Job drawing, mm, ordinate dimensions from the low corner. One solid piece. Coordinates: 2 decimals unless noted, no trailing zeros. Write each loop counter-clockwise with the first axis right and the second up, starting at its lowest first coordinate (ties: lowest second). Pieces come first, ordered by that corner, then holes.
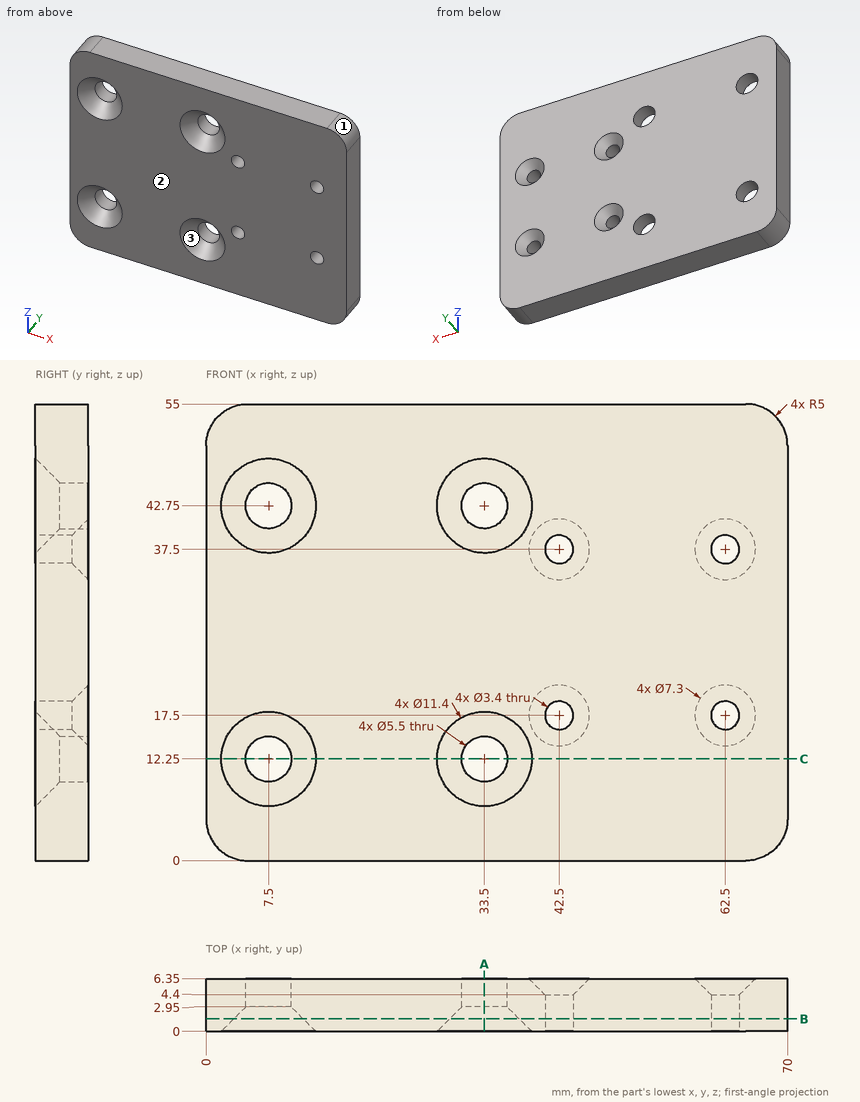
1. Saw through at C-C on z = 12.25. List the corners of the cut face in (x, y), plus the area to 3 significant figures.
Computed values:
outline: (0, 0) - (1.8, 0) - (4.75, 2.95) - (4.75, 6.35) - (0, 6.35) - close; (10.25, 2.95) - (13.2, 0) - (27.8, 0) - (30.75, 2.95) - (30.75, 6.35) - (10.25, 6.35) - close; (36.25, 2.95) - (39.2, 0) - (70, 0) - (70, 6.35) - (36.25, 6.35) - close
area: 357 mm2
2. Saw through at B-B on y = 1.5. State how many separate pieces and enclosed holes the cut face has, plus the area to 3 significant figures.
Computed values:
separate pieces: 1
enclosed holes: 8
area: 3,570 mm2
3. Flat gauge pins, fed straight in: pin 1 (4.5 mm diameter, centred on x = 42.5, z = 17.5, fed in from +Y); pin 2 (5.5 mm diameter, centred on x = 42.5, z = 37.5, fed in from +Y). Where does each tip first touch, or does it go through?
Computed values:
pin 1: stops at y = 4.95
pin 2: stops at y = 5.45
4. Mould opens along Z. For the marked faces 1, 2 and 3 say: +Z half, -Z half, draft (parallel to the pull), parting line (faces both ways), or undercut.
Computed values:
face 1: +Z half
face 2: draft
face 3: undercut
5. Saw through at A-A on x = 33.5. List the corners of the cut face in (y, z), plus the area to 3 significant figures.
Computed values:
outline: (0, 0) - (6.35, 0) - (6.35, 9.5) - (2.95, 9.5) - (0, 6.55) - close; (0, 17.95) - (2.95, 15) - (6.35, 15) - (6.35, 40) - (2.95, 40) - (0, 37.05) - close; (0, 48.45) - (2.95, 45.5) - (6.35, 45.5) - (6.35, 55) - (0, 55) - close
area: 262 mm2
6. Probe line 1 along X through (y, z) = (3.4, 37.5); line 2 along Z through (x, y) = (33.5, 5); line 3 along Z through (x, y) = (62.5, 2.9). List the from-to ranges inside material, lowest first.
Computed values:
line 1: x = 0 to 40.8, 44.2 to 60.8, 64.2 to 70
line 2: z = 0 to 9.5, 15 to 40, 45.5 to 55
line 3: z = 0 to 15.8, 19.2 to 35.8, 39.2 to 55
